For this review, take the finished solid that the model builds, in its own axes (mm). Face numbers are marked on the shaded views. A direction names the side the tool comes from. Give positions to 0.01 mm unless a question says otherwise; leave off trailing zeros. Order: outer loops, then holes, each group sorted by start corner. A loop starts at its lowest first (then second) coordinate and runs counter-clockwise, first axis right, second up. Notation, with made-up numbers: (19, 39) -> (34, 39) arc R17 ccw to (34, 66) -> close; hole circle Ø10 at (-25.75, 83.25). An arc over 180 degrees is marked (long way). One line per item, written item: value. Start each with the question number.
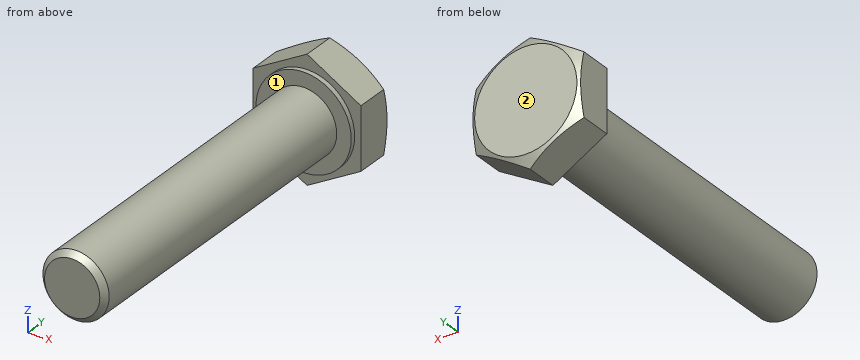
Autodesk Inventor part; units mm, degrees
ref_plane "YZ Plane" through (0, 0, 0) normal (1, 0, 0) x (0, 1, 0)
ref_plane "XZ Plane" through (0, 0, 0) normal (0, 1, 0) x (-1, 0, 0)
ref_plane "XY Plane" through (0, 0, 0) normal (0, 0, 1) x (1, 0, 0)
sketch "Sketch1" plane through (0, 0, 0) normal (0, 0, 1) x (1, 0, 0)
  line L0 (0, 0) -> (6.175, 0)
  line L1 (9.75, -2.064) -> (9.75, -4.7)
  line L2 (5.75, -5.3) -> (4, -5.3)
  line L3 (4, -5.3) -> (4, -45.3)
  line L4 (4, -45.3) -> (0, -45.3)
  line L5 (0, -45.3) -> (0, 0)
  line L6 (5.75, -5.3) -> (5.75, -4.7)
  line L7 (5.75, -4.7) -> (9.75, -4.7)
  line L8 (6.175, 0) -> (9.75, -2.064)
  dimension "d0" = 19.5
  dimension "d1" = 8
  dimension "d3" = 40
  dimension "d4" = 11.5
  dimension "d5" = 0.6
  dimension "d22" = 30
  dimension "d23" = 12.35
  dimension "d24" = 5.3
revolve "Revolution1" add sketch "Sketch1" angle 360 about axis through (0, -45.3, 0) along (0, 1, 0)
sketch "Sketch2" plane through (0, 0, 0) normal (0, 1, 0) x (1, 0, 0)
  line L0 (0, -7.5056) -> (-6.5, -3.7528)
  line L1 (-6.5, -3.7528) -> (-6.5, 3.7528)
  line L2 (-6.5, 3.7528) -> (0, 7.5056)
  line L3 (0, 7.5056) -> (6.5, 3.7528)
  line L4 (6.5, 3.7528) -> (6.5, -3.7528)
  line L5 (6.5, -3.7528) -> (0, -7.5056)
  circle A0 centre (0, 0) radius 9.75
  point P0 (0, 0)
  point P1 (0, 0)
  dimension "d25" = 13
extrude "Extrusion1" cut sketch "Sketch2" against normal blind 5.3
thread "Thread1"
chamfer "Chamfer1" distance 0.6667 angle 45 1 edges at (-4, -45.3, 0)
equation "\"d0\" = 1.5 * S_"
equation "\"d1\" = d1_"
equation "\"d3\" = L"
equation "\"d4\" = dw"
equation "\"d5\" = hw"
equation "\"d23\" = 0.95 * S_"
equation "\"d24\" = k"
equation "\"d14\" = b"
equation "\"d16\" = 0.0833333 * d"
equation "\"d25\" = S_"
equation "\"d26\" = k"
equation "\"d\" = 8"
equation "\"d1_\" = 8"
equation "\"S_\" = 13"
equation "\"k\" = 5.3"
equation "\"e\" = 14.2"
equation "\"L\" = 40"
equation "\"b\" = 22"
equation "\"Grip_Length\" = 18"
equation "\"dw\" = 11.5"
equation "\"hw\" = 0.6"
properties part number "Bolt A M8-6g×40(S13) GOST 7798-70" material "Steel, Mild"
Q1. For the marked faces 1 and 2, list the 3-axis set-ups (+Z, -Z, +X, -X, +Y, -Y) from which the entire face can be reached by the end or side of a thin tool; tool diameter is ignored.
Q2. Take a section at A-A (z = 0). State the section outline as (x, y) points (3 decimals).
Q3. For pin 1 Ø6 at (y, z) = (-20, 0) entering from +X; pin 2 Ø2 at (x, y) = (-4, -11.5) entering from +Z; pin 3 Ø1.5 at (y, z) = (-20, 3) entering from -X, all flat-tipped, find the tip position at first contact; note any pin that passes through.
Q4. For line 1 along Y through (x, z) = (-2.25, -5.25); line 2 along Y through (x, z) = (-0.5, 6); line 3 along Z through (x, y) = (2.75, -32), list the stretches that pass through material, from the lowest coordinate up.
Q5. Take a section at B-B (y = -34.5). State the section outline as (x, z) points, and give its area (3 significant figures).
Answers below:
1. face 1: -Y
1. face 2: +Z, -Z, +X, -X, +Y
2. outline: (-6.5, -4.7) -> (-5.75, -4.7) -> (-5.75, -5.3) -> (-4, -5.3) -> (-4, -44.633) -> (-3.333, -45.3) -> (3.333, -45.3) -> (4, -44.633) -> (4, -5.3) -> (5.75, -5.3) -> (5.75, -4.7) -> (6.5, -4.7) -> (6.5, -0.188) -> (6.175, 0) -> (-6.175, 0) -> (-6.5, -0.188) -> close
3. pin 1: stops at x = 4
3. pin 2: stops at z = 2.65
3. pin 3: stops at x = -3.31
4. line 1: y = -5.3 to 0
4. line 2: y = -4.7 to 0
4. line 3: z = -2.9 to 2.9
5. outline: circle Ø8 at (0, 0)
5. area: 50.3 mm²
